The listing builds one solid part. Answer for the finished solid, in the listing's coordinates (mm). A direction names the side the tool comes from. Give positions to 0.01 mm unless a question says otherwise; leave off trailing zeros. Write each loop counter-clockwise with the first axis right and the second up, starting at its lowest first coordinate (ties: lowest second). Pieces come first, ordered by that corner, then holes. Notation, with made-up numbers: M 51,-12.75 L 73,-12.75 A27 cw 73,13.25 Z; hole C -40,17 d10. An arc over 180 degrees is marked long. Answer as a JSON object with one key per item and string values.
```python
from build123d import *

# Parameters (mm, degrees)
F1_DEPTH    = 8
F3_D        = 5.5
F4_SIZE     = 0.5
F5_T1_DEPTH = 17.2867319519


# Not quite as in the source:
# - a fillet or chamfer that OpenCascade refuses, or shapes differently, is made with other operations: its cross-section is extruded or revolved along the edge and cut away or added


with BuildPart() as f1:
    # F0 (on Front) → F1 (new body)
    with BuildSketch(Plane.XZ):
        Polygon((150, 180), (70, 180), (70, 80), (45, 40), (0, 40), (0, 0), (125, 0), (125, 40), (150, 80), align=None)
    extrude(amount=F1_DEPTH)

    # F3 (through all)
    with Locations(Plane.XZ.offset(8)):
        with Locations((93, 34), (6, 34), (32, 34), (119, 34), (119, 6), (93, 6), (32, 6), (6, 6)):
            Hole(F3_D / 2)

    # F4
    f4_edges = [f1.edges().sort_by_distance(p)[0] for p in [
        (110, -8, 180),
        (70, -8, 130),
        (57.5, -8, 60),
        (22.5, -8, 40),
        (0, -8, 20),
        (62.5, -8, 0),
        (125, -8, 20),
        (137.5, -8, 60),
        (150, -8, 130),
        (110, 0, 180),
        (150, 0, 130),
        (137.5, 0, 60),
        (125, 0, 20),
        (0, 0, 20),
        (22.5, 0, 40),
        (57.5, 0, 60),
        (70, 0, 130),
    ]]
    chamfer(f4_edges, length=F4_SIZE)

    # F5: chamfer of 2 on 5 edges, made by hand

    # F5_s2 → F5_t1 (cut)
    with BuildSketch(Plane.XZ.offset(-4.6433659759)):
        Polygon((72, 180), (70, 178), (70, 180), align=None)
        Polygon((148, 180), (150, 178), (150, 180), align=None)
        Polygon((2, 40), (0, 38), (0, 40), align=None)
        Polygon((2, 0), (0, 2), (0, 0), align=None)
        Polygon((125, 2), (123, 0), (125, 0), align=None)
    extrude(amount=F5_T1_DEPTH, mode=Mode.SUBTRACT)


solid = f1.part
```
1. For faces 1 (the flat face through (70, -4, 130)), 2 (the flat face through (125, -4, 21)), 3 (the flat face through (91, -8, 91)), determine the directions among +Z, -Z, +X, -X, +Y, -Y from which every point of the face is accessible in a straight line to the end or side of a thin tool.
Verdict:
{"face 1": "+Z, -X, +Y, -Y", "face 2": "-Z, +X, +Y, -Y", "face 3": "+Z, -Z, +X, -X, -Y"}
2. The mould has two halves that part along Z. Classify faces 4 (the cylindrical face through (119.358, -3.944, 36.727)), 5 (the flat face through (24, -4, 40)), 6 (the flat face through (0, -4, 20)), 7 (the flat face through (137.077, -0.253, 59.789)): released by +Z, released by -Z, zero draft, split by the parting line, or undercut.
Verdict:
{"face 4": "undercut", "face 5": "released by +Z", "face 6": "zero draft", "face 7": "released by -Z"}
3. A cutting plane is placed at C-C, the plane y = -3.5. Count the separate pieces of the cut face and the enclosed holes in it, plus the area to 3 significant figures.
Verdict:
{"separate pieces": "1", "enclosed holes": "8", "area": "16,000 mm2"}
4. Flat-ended cylindrical pins translate along their axes: pin 1 (3 mm diameter, centred on y = -1, z = 96.5, fed in from -X); pin 2 (1.5 mm diameter, centred on x = 38, y = -1, fed in from +Z); pin 3 (3.5 mm diameter, centred on y = -5, z = 15.5, fed in from +X). Find the tip coordinate at first contact, or state that the pin passes through.
Verdict:
{"pin 1": "stops at x = 70", "pin 2": "stops at z = 40", "pin 3": "stops at x = 125"}
5. A cutting plane is placed at A-A, the plane z = 6. Give the vertices of the cut face in (x, y), plus the area to 4 significant figures.
Verdict:
{"outline": "M 0,-7.5 L 0.5,-8 L 3.25,-8 L 3.25,0 L 0.5,0 L 0,-0.5 Z; M 8.75,-8 L 29.25,-8 L 29.25,0 L 8.75,0 Z; M 34.75,-8 L 90.25,-8 L 90.25,0 L 34.75,0 Z; M 95.75,-8 L 116.25,-8 L 116.25,0 L 95.75,0 Z; M 121.75,-8 L 124.5,-8 L 125,-7.5 L 125,-0.5 L 124.5,0 L 121.75,0 Z", "area": "823.5 mm2"}
6. A cutting plane is placed at D-D, the plane z = 168. Give the vertices of the cut face in (x, y).
Verdict:
{"outline": "M 70,-7.5 L 70.5,-8 L 149.5,-8 L 150,-7.5 L 150,-0.5 L 149.5,0 L 70.5,0 L 70,-0.5 Z"}
7. A cutting plane is placed at B-B, the plane x = 32. Give the vertices of the cut face in (y, z).
Verdict:
{"outline": "M -8,0.5 L -7.5,0 L 0,0 L 0,3.25 L -8,3.25 Z; M -8,8.75 L 0,8.75 L 0,31.25 L -8,31.25 Z; M -8,36.75 L 0,36.75 L 0,39.5 L -0.5,40 L -7.5,40 L -8,39.5 Z"}
8. Consider line 1 along Z through (x, y) = (6, -3.25); line 2 along Z through (x, y) = (93, -4.5); line 3 along X through (y, z) = (-2.25, 152). Determine where each line is inside the solid, lowest interval first.
Verdict:
{"line 1": "z = 0 to 3.25, 8.75 to 31.25, 36.75 to 40", "line 2": "z = 0 to 3.25, 8.75 to 31.25, 36.75 to 180", "line 3": "x = 70 to 150"}
